Work out the finished part from the listing and answer in its coordinate system (mm). Face numbers are marked on the shaded views. A direction names the side the tool comes from. Coordinates: 2 decimals unless noted, no trailing zeros. Write each loop counter-clockwise with the first axis right and the second up, starting at its lowest first coordinate (ties: lowest second). Pieces come first, ordered by that corner, then holes. Notation, with made-up numbers: (44, 43.5) - (52, 43.5) arc R14 ccw to (52, 48.5) - close; hole circle Ø9 at (83, 72). An arc over 180 degrees is marked (long way). Use one line per item in the form item = value. Start each with the question number.
Item 1: A cutting plane is placed at D-D (x = -6.75). Write down the section's boundary in (y, z), then the cut area to 3 significant figures.
Item 2: Determine the mould class of the marked faces 6, 7 and 8 for opening direction Y: released by +Y, released by -Y, zero draft, split by the parting line, or undercut.
Item 3: A cutting plane is placed at B-B (y = 8.5). Write down the section's boundary in (x, z).
Item 4: Consider probe 1 along Y at (x, z) = (-7, 1.25); probe 2 along X at (y, z) = (7, 2.4); probe 3 along Y at (x, z) = (-7.5, 2.25). Determine where each line is inside the solid, lowest interval first.
Item 5: Given pin 1 (1.5 mm diameter, centred on x = -4, z = 4, fed in from +Y); pin 2 (0.6 mm diameter, centred on x = -11.5, y = 0.5, fed in from +Z); pin 3 (1.5 mm diameter, centred on y = 1, z = 5, fed in from -X), each flat-ended and moving along its own axis, determine where each tip first touches the part or whether it passes through.
Item 6: A cutting plane is placed at A-A (z = 7.5). Write down the section's boundary in (x, y), then the cut area to 3 significant figures.
Item 7: For the marked faces 1, 2, 3, 4 and 5, determine the directions among +Z, -Z, +X, -X, +Y, -Y from which every point of the face is accessible in a straight line to the end or side of a thin tool.
Item 8: A cutting plane is placed at C-C (z = 2.75). Write down the section's boundary in (x, y), then the cut area to 3 significant figures.
from build123d import *

# Parameters (mm, degrees)
BOSS_EXTRUDE1_DEPTH    = 14
CUT_EXTRUDE1_START     = -8
CUT_EXTRUDE1_OUTLINE_R = 2
CUT_EXTRUDE1_DEPTH     = 8
CUT_EXTRUDE2_DEPTH     = 2


# Read off the part's stored shape, not the designer's step: Cut-Extrude1
with BuildPart() as part:
    # Sketch2 → Boss-Extrude1 (new body)
    with BuildSketch(Plane(origin=(0, 0, 0), x_dir=(0, 0, -1), z_dir=(1, 0, 0))):
        Polygon((0, 0), (0, 7), (-1, 7), (-1, 10), (-3, 10), (-3, 7), (-5, 7), (-5, 4), (-8, 4), (-8, 2), (-7, 2), (-7, 0), align=None)
    extrude(amount=-BOSS_EXTRUDE1_DEPTH)

    # Cut-Extrude1 outline → Cut-Extrude1 (cut)
    with BuildSketch(Plane.XY.offset(8).offset(CUT_EXTRUDE1_START)):
        with BuildLine():
            Line((-14, 0), (-9.828427125, 8))
            ThreePointArc((-9.828427125, 8), (-8.732050808, 9.449489743), (-7, 10))
            Line((-7, 10), (-14, 10))
            Line((-14, 10), (-14, 0))
        make_face()
        Polygon((-5, 2), (-9, 2), (-8, 0), (-6, 0), align=None)
        with BuildLine():
            Line((0, 0), (0, 10))
            Line((0, 10), (-7, 10))
            ThreePointArc((-7, 10), (-5.267949192, 9.449489743), (-4.171572875, 8))
            Line((-4.171572875, 8), (0, 0))
        make_face()
        with Locations((-7, 7)):
            Circle(CUT_EXTRUDE1_OUTLINE_R)
    extrude(amount=CUT_EXTRUDE1_DEPTH, mode=Mode.SUBTRACT)

    # Sketch4 → Cut-Extrude2 (cut)
    with BuildSketch(Plane.XY.offset(8)):
        Polygon((-9.914213562, 4), (-9.042893219, 2), (-5.042893219, 2), (-4.085786438, 4), align=None)
    extrude(amount=-CUT_EXTRUDE2_DEPTH, mode=Mode.SUBTRACT)


solid = part.part
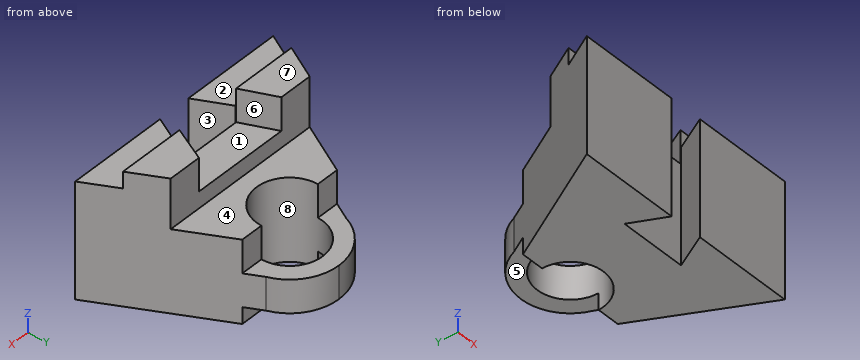
Answer:
q1.outline = (2, 0) - (5.02, 0) - (5.02, 5) - (4, 5) - (4, 6) - (2, 6) - close; (8.98, 1) - (9.99, 1) - (9.99, 3) - (8.98, 3) - close
q1.area = 19.1 mm²
q2.face_6 = released by +Y
q2.face_7 = zero draft
q2.face_8 = undercut
q3.outline = (-9.6, 1) - (-8.32, 1) - (-8.32, 3) - (-9.6, 3) - close; (-5.68, 1) - (-4.4, 1) - (-4.4, 3) - (-5.68, 3) - close
q4.probe_1 = 2 to 5, 9 to 10
q4.probe_2 = -10.35 to -9, -5 to -3.65
q4.probe_3 = 2 to 5.06, 8.94 to 9.96
q5.pin_1 = 7
q5.pin_2 = 7
q5.pin_3 = -13.87
q6.outline = (-12.96, 2) - (-9.04, 2) - (-9.91, 4) - (-11.91, 4) - close; (-5.04, 2) - (-1.04, 2) - (-2.09, 4) - (-4.09, 4) - close
q6.area = 11.9 mm²
q7.face_1 = +Z, +Y
q7.face_2 = +Z, +X, -X, -Y
q7.face_3 = +Z, -Z
q7.face_4 = +Z, +X, -X, +Y
q7.face_5 = -Z, +X, -X, +Y
q8.outline = (-14, 0) - (-8, 0) - (-9, 2) - (-5, 2) - (-6, 0) - (0, 0) - (-4.17, 8) arc R3 ccw to (-9.83, 8) - close; hole circle Ø4 at (-7, 7)
q8.area = 68.3 mm²
